from build123d import *

# Parameters (mm, degrees)
SKETCH1_W           = 126
SKETCH1_H           = 66
SKETCH1_W_2         = 120
SKETCH1_H_2         = 60
EXTRUDE_THIN1_DEPTH = 600
SKETCH2_W           = 120
SKETCH2_H           = 60
BOSS_EXTRUDE1_DEPTH = 3


with BuildPart() as part:
    # Sketch1 → Extrude-Thin1 (new, symmetric)
    with BuildSketch(Plane(origin=(0, 0, 0), x_dir=(1, 0, 0), z_dir=(0, 1, 0))):
        Rectangle(SKETCH1_W, SKETCH1_H)
        Rectangle(SKETCH1_W_2, SKETCH1_H_2, mode=Mode.SUBTRACT)
    extrude(amount=EXTRUDE_THIN1_DEPTH, both=True)

    # Sketch2 → Boss-Extrude1 (add)
    with BuildSketch(Plane(origin=(0, 600, 0), x_dir=(1, 0, 0), z_dir=(0, 1, 0))):
        Rectangle(SKETCH2_W, SKETCH2_H)
    extrude(amount=-BOSS_EXTRUDE1_DEPTH)


solid = part.part
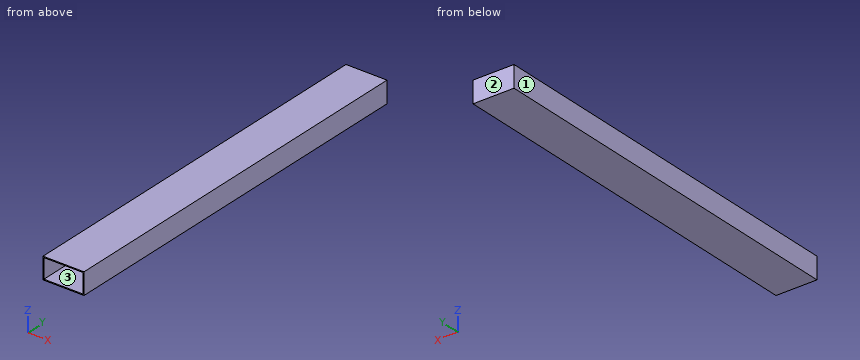
Model file for the job. Use its own axes, mm. Face numbers are marked on the shaded views. Coordinates: 2 decimals unless noted, no trailing zeros. Order: outer loops, then holes, each group sorted by start corner. A loop starts at its lowest first (then second) coordinate and runs counter-clockwise, first axis right, second up. Notation, with made-up numbers: (74.5, 65) -> (118.5, 65) arc R27 cw to (118.5, 83) -> close; hole circle Ø1 at (-9.5, 57.25). An arc over 180 degrees is marked (long way). Return JSON: item names as keys, results as strings. Group by question number.
Item 1: Saw through at B-B on z = 15. Write the cut outline in (x, y), then the cut area to 3 significant figures.
Item 2: Flat gauge pin, fed straight in: P1, Ø18, axis at x = -14.5, z = 7.5, coming from the -Y side. Where does the tip first touch, or does it go through?
Item 3: Saw through at A-A on y = -187. Write the cut outline in (x, z).
Item 4: Saw through at C-C on x = -11. Write the cut outline in (y, z).
Item 5: Wall check: line 1 along Z through (x, y) = (56, -447); line 2 along X through (y, z) = (113.5, 26); line 3 along Y through (x, z) = (-12.5, 0). Give the ranges that are in metal, low to high. Write a range as [from, to].
Item 6: Pull direction X, two halves, no side cores. Call the marked faces 1, 2 and 3: pulls with the +X half, pulls with the -X half, needs draft (parallel to the pull), parting line crosses it, or undercut.
Values found:
{
 "1": {"outline": "(-63, -600) -> (-60, -600) -> (-60, 597) -> (60, 597) -> (60, -600) -> (63, -600) -> (63, 600) -> (-63, 600) -> close", "area": "7,560 mm2"},
 "2": {"P1": "stops at y = 597"},
 "3": {"outline": "(-63, -33) -> (63, -33) -> (63, 33) -> (-63, 33) -> close; hole (-60, -30) -> (60, -30) -> (60, 30) -> (-60, 30) -> close"},
 "4": {"outline": "(-600, -33) -> (600, -33) -> (600, 33) -> (-600, 33) -> (-600, 30) -> (597, 30) -> (597, -30) -> (-600, -30) -> close"},
 "5": {"line 1": "z = [-33, -30], [30, 33]", "line 2": "x = [-63, -60], [60, 63]", "line 3": "y = [597, 600]"},
 "6": {"face 1": "pulls with the -X half", "face 2": "needs draft", "face 3": "undercut"}
}
